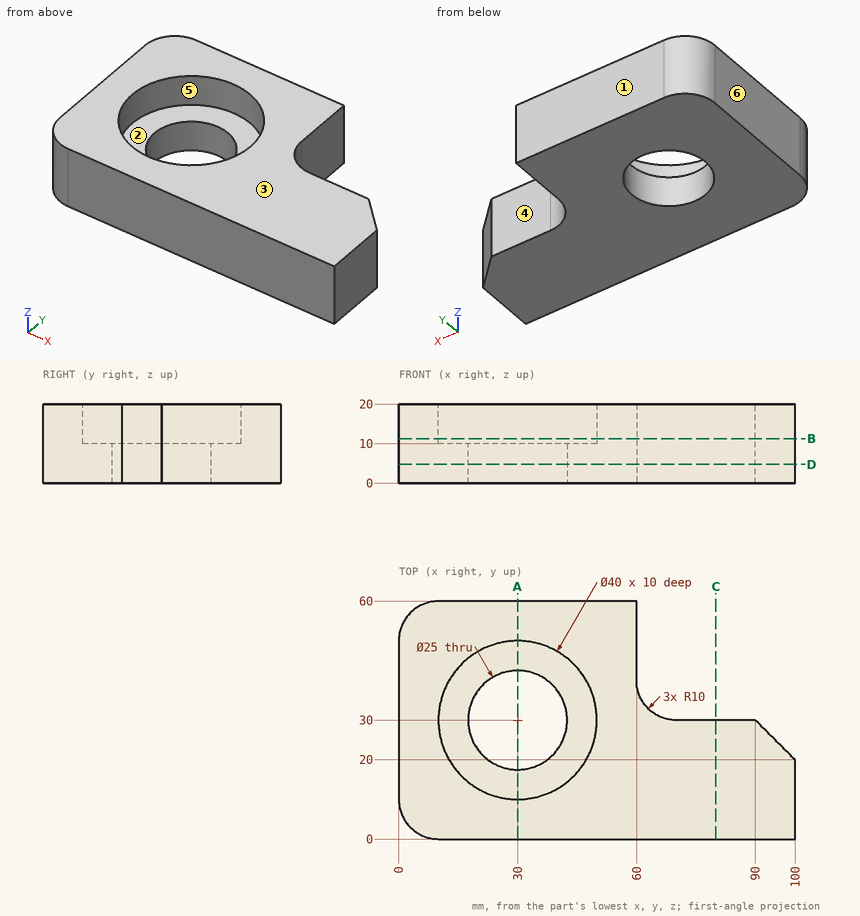
Could you check a few things on this drawing? It's one solid part, dimensions in mm from its lowest x, y, z. A direction names the side the tool comes from. Give positions to 0.01 mm unless a question says otherwise; leave off trailing zeros. Write each loop counter-clockwise with the first axis right and the second up, starting at its lowest first coordinate (ties: lowest second). Pieces come first, ordered by that corner, then holes. Notation, with made-up numbers: (16.25, 84.5) - (50.25, 84.5) arc R21 cw to (50.25, 118.5) - close; hole circle Ø2 at (85.25, -15.5). An arc over 180 degrees is marked (long way). Use CSV: the item, a comma, the result in double quotes. Start each with the question number.
Item 1: I want a section at D-D, the plane z = 4.75. Please give me the cut outline in (x, y).
Item 2: I want a section at B-B, the plane z = 11.25. Please give me the cut outline in (x, y).
Item 3: I want a section at C-C, the plane x = 80. Please give me the cut outline in (y, z).
Item 4: If I drill on line 1 along Y through (x, z) = (30, 4); line 2 along Y through (x, z) = (30, 16.25); line 3 along X through (y, z) = (27, 5), over which ranges is the centre line in solid material (lowest first)?
Item 5: I'm going to push flat-ended pins straight in: pin 1 (10 mm diameter, centred on y = 46, z = 8, fed in from +X); pin 2 (3 mm diameter, centred on x = 69, z = 6, fed in from +Y); pin 3 (6 mm diameter, centred on x = 83, z = 10, fed in from +Y). Where does each tip first touch, or does it pass through?
Item 6: If we mould it in two halves opening along Y, with no side actions, what happens to the marked faces 1, 2 and 3? For each: pulls with the +Y half, pulls with the -Y half, needs draft (parallel to the pull), parting line crosses it, or undercut.
Item 7: For the marked faces 4, 5 and 6, which set-ups out of +Z, -Z, +X, -X, +Y, -Y let a thin tool reach every point of the face, with its end or its side?
Item 8: I want a section at A-A, the plane x = 30. Please give me the cut outline in (y, z).
Findings:
1,outline,"(0, 10) arc R10 ccw to (10, 0) - (100, 0) - (100, 20) - (90, 30) - (70, 30) arc R10 cw to (60, 40) - (60, 60) - (10, 60) arc R10 ccw to (0, 50) - close; hole circle Ø25 at (30, 30)"
2,outline,"(0, 10) arc R10 ccw to (10, 0) - (100, 0) - (100, 20) - (90, 30) - (70, 30) arc R10 cw to (60, 40) - (60, 60) - (10, 60) arc R10 ccw to (0, 50) - close; hole circle Ø40 at (30, 30)"
3,outline,"(0, 0) - (30, 0) - (30, 20) - (0, 20) - close"
4,line 1,"y = 0 to 17.5, 42.5 to 60"
4,line 2,"y = 0 to 10, 50 to 60"
4,line 3,"x = 0 to 17.87, 42.13 to 93"
5,pin 1,"stops at x = 60"
5,pin 2,"stops at y = 30.32"
5,pin 3,"stops at y = 30"
6,face 1,"pulls with the +Y half"
6,face 2,"undercut"
6,face 3,"needs draft"
7,face 4,"+Z, -Z, +X, +Y"
7,face 5,"+Z"
7,face 6,"+Z, -Z, -X, +Y, -Y"
8,outline,"(0, 0) - (17.5, 0) - (17.5, 10) - (10, 10) - (10, 20) - (0, 20) - close; (42.5, 0) - (60, 0) - (60, 20) - (50, 20) - (50, 10) - (42.5, 10) - close"
